Geometry check sheet. Reference: drawing and pictorial views, mm from the part's lowest x, y, z. A direction names the side the tool comes from. Round coordinates to 2 decimals unless told otherwise and drop trailing zeros. Loops run counter-clockwise (first coordinate to the right, second up) from the corner with the lowest first, then second, coordinate; pieces in that order, holes last. Notation, with made-up numbers: (83, 45) - (137, 45) arc R24 ccw to (137, 64) - close; hole circle Ø10 at (9, -23.75). An arc over 180 degrees is marked (long way). Put each result on its own line as item: value. Start each with the question number.
Item 1: Section check C-C, the plane x = 10.5. Record the cut outline in (y, z).
Item 2: Draft check along X on the marked faces 1, 2, 3 and 4. Enter one of: pulls with the +X half, pulls with the -X half, needs draft (parallel to the pull), parting line crosses it, or undercut.
Item 3: Gauge pin test, flat ends, axial feed: pin 1 Ø5.5 at (x, y) = (14.5, 4) entering from +Z; pin 2 Ø3 at (x, z) = (13, 17) entering from -Y; pin 3 Ø5 at (y, z) = (6.5, 15.5) entering from +X. Record the tip position at first contact, or that the pin passes through.
Item 4: Tool access check on the marked faces 5, 6, 7, 8 and 9. Record the directions out of +Z, -Z, +X, -X, +Y, -Y that give a thin tool (end or side, any length) a straight path to the whole face; none if there is none.
Item 5: Material ranges on line 1 along Y through (x, z) = (13, 3.8); line 2 along Y through (x, z) = (13, 1); line 3 along X through (y, z) = (22.5, 20), recorded low to high.
Item 6: Section check A-A, the plane y = 6. Record the cut outline in (x, z), and give its area (4 significant figures).
Item 7: Section check B-B, the plane z = 4. Record the cut outline in (x, y).
Item 8: Section check D-D, the plane z = 8.5. Record the cut outline in (x, y).
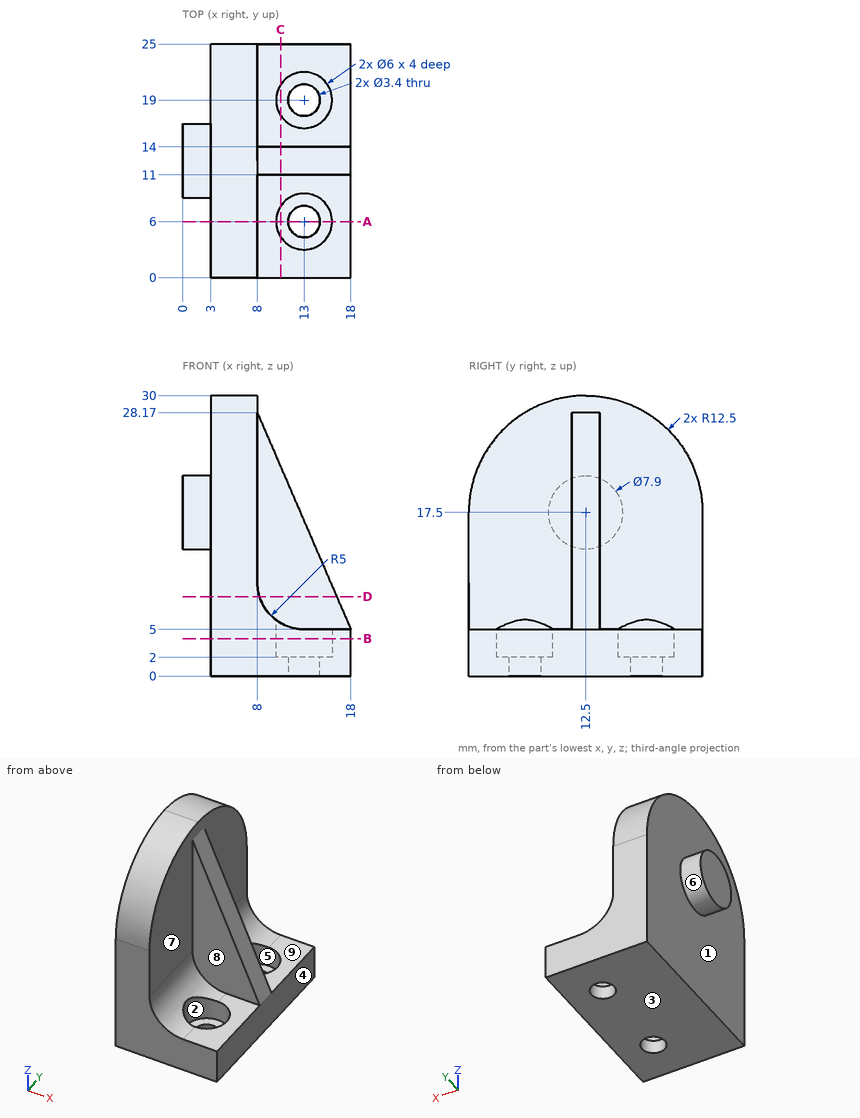
Check result:
1. outline: (0, 0) - (25, 0) - (25, 5.67) - (20.66, 5.67) - (20.66, 2) - (17.34, 2) - (17.34, 5.67) - (14, 5.67) - (14, 22.38) - (11, 22.38) - (11, 5.67) - (7.66, 5.67) - (7.66, 2) - (4.34, 2) - (4.34, 5.67) - (0, 5.67) - close
2. face 1: pulls with the -X half
2. face 2: undercut
2. face 3: needs draft
2. face 4: pulls with the +X half
3. pin 1: z = 5.13
3. pin 2: y = 11
3. pin 3: x = 8
4. face 5: +Z
4. face 6: -X
4. face 7: +Z, +X
4. face 8: +Z, +X, -Y
4. face 9: +Z, +X, +Y
5. line 1: 0 to 3, 9 to 16, 22 to 25
5. line 2: 0 to 4.3, 7.7 to 17.3, 20.7 to 25
5. line 3: 3 to 8
6. outline: (3, 0) - (11.3, 0) - (11.3, 2) - (10, 2) - (10, 6) arc R5 cw to (8, 10) - (8, 28.18) - (3, 28.18) - close; (14.7, 0) - (18, 0) - (18, 5) - (16, 5) - (16, 2) - (14.7, 2) - close
6. area: 170.5 mm²
7. outline: (3, 0) - (18, 0) - (18, 25) - (3, 25) - close; hole circle Ø6 at (13, 6); hole circle Ø6 at (13, 19)
8. outline: (3, 0) - (8.23, 0) - (8.23, 11) - (16.49, 11) - (16.49, 14) - (8.23, 14) - (8.23, 25) - (3, 25) - close
